Part model, mm, in its own coordinate system. A direction names the side the tool comes from. Give positions to 0.01 mm unless a question says otherwise; leave off trailing zeros. Write each loop counter-clockwise with the first axis right and the second up, starting at its lowest first coordinate (ties: lowest second). Pieces come first, ordered by that corner, then holes. Notation, with made-up numbers: (4.5, 42) - (35.5, 42) arc R18 ccw to (35.5, 67) - close; hole circle Ø3 at (12.25, -6.5). An arc over 180 degrees is marked (long way). Answer as a JSON object with one key per item and string values. Group by question number.
Autodesk Inventor part; units mm, degrees
ref_plane "YZ Plane" through (0, 0, 0) normal (1, 0, 0) x (0, 1, 0)
ref_plane "XZ Plane" through (0, 0, 0) normal (0, 1, 0) x (-1, 0, 0)
ref_plane "XY Plane" through (0, 0, 0) normal (0, 0, 1) x (1, 0, 0)
sketch "Skizze1" plane through (0, 0, 0) normal (0, 1, 0) x (-1, 0, 0)
  line L0 (6.8592, -116.2444) -> (0.8592, -116.2444)
  line L1 (0.8592, -116.2444) -> (0.8592, 8.7556)
  line L2 (6.8592, 8.7556) -> (6.8592, -116.2444)
  line L3 (7.8592, -116.2444) -> (-0.1408, -116.2444)
  line L4 (-0.1408, -116.2444) -> (-0.1408, -106.2444)
  line L5 (-0.1408, -106.2444) -> (7.8592, -106.2444)
  line L6 (7.8592, -106.2444) -> (7.8592, -116.2444)
  line L7 (3.8592, 157.3916) -> (3.8592, -262.6084)
  line L8 (6.8592, 8.7556) -> (0.8592, 8.7556)
  point P0 (0, 0)
  point P1 (0.8592, -106.2444)
  point P2 (6.8592, -106.2444)
  point P3 (6.8592, -116.2444)
  point P4 (3.8592, -116.2444)
  dimension "d1" = 125
  dimension "d9" = 6
  dimension "d25" = 8
  dimension "d26" = 10
  dimension "d27" = 1
extrude "Extrusion1" add sketch "Skizze1" along normal blind 3
sketch "Skizze2" plane through (0, 3, 0) normal (0, 1, 0) x (1, 0, 0)
  line L0 (-3.8592, 111.2444) -> (-6.8592, 111.2444) construction
  line L1 (-3.8592, 111.2444) -> (-0.8592, 111.2444) construction
  line L2 (-0.8592, -8.7556) -> (-0.8592, 106.2444) construction
  line L3 (-6.8592, 106.2444) -> (-6.8592, -8.7556) construction
  line L4 (0.1408, 116.2444) -> (-7.8592, 116.2444)
  point P0 (0, 0)
  point P1 (-0.8592, 16.2444)
  point P2 (-6.8592, 16.2444)
  dimension "d28" = 5
hole "Bohrung1" at (-3.8592, 3, -111.2444) direction (0, -1, 0) diameter 2.459 end through all
sketch "Skizze3" plane through (0.1408, 0, -116.2444) normal (0, 0, -1) x (-1, 0, 0)
  line L0 (4, 0) -> (4, 0.7)
  circle A0 centre (4, 0.7) radius 1.5
  line L1 (0, 0) -> (8, 0)
  point P0 (0.1408, 0)
  dimension "d29" = 3
  dimension "d30" = 0.7
extrude "Extrusion2" add sketch "Skizze3" along normal blind 3
sketch "Skizze4" plane through (0, 0, 0) normal (0, -1, 0) x (1, 0, 0)
  line L0 (-0.8592, 8.7556) -> (-0.8592, -106.2444)
  line L1 (-6.8592, -69.2444) -> (-0.8592, -69.2444)
  line L2 (-0.8592, -69.2444) -> (-0.8592, -29.2444)
  line L3 (-0.8592, -29.2444) -> (-6.8592, -29.2444)
  line L4 (-6.8592, -29.2444) -> (-6.8592, -69.2444)
  point P0 (0, 0)
  point P1 (-0.8592, -69.2444)
  point P2 (-6.8592, -106.2444)
  dimension "d34" = 40
  dimension "d37" = 37
  dimension "d38" = 6
extrude "Extrusion3" add sketch "Skizze4" along normal blind 6
chamfer "Fasen1" distance 40 distance2 4 1 edges at (-3.8592, -6, -29.2444) measured on face at (-4.8592, -6, -42.5778)
properties part number "SchubstangeA" material "PC/ABS-Kunststoff, 3DDruck, PLA"
1) Drop flat-ended pins along their axis: P1, Ø0.6, axis at x = -4.5, y = -1, coming from the +Z side; P2, Ø2, axis at x = -4.5, z = -59, coming from the -Y side; P3, Ø1, axis at x = -1.5, z = -16, coming from the -Y side. Give the stop position or say it passes through.
2) Two-plate mould, pull along Z, no slides. Class faces 5 (the flat face through (-4, 0, -92)), 6 (the flat face through (-4, -1, -29.244)), 7 (the cylindrical face through (-3.913, 1.479, -112.473)), 8 (the flat face through (-0.859, 0, -50)): +Z half, -Z half, draft (parallel to the pull), parting line (faces both ways), or undercut.
3) Which spindle directions (+Z, -Z, +X, -X, +Y, -Y) get a long thin tool onto all of the face, cutting with end or side? Do faces 1 (the flat face through (-7.859, 1, -111)), 2 (the cylindrical face through (-2.36, 0.63, -117.72)), 3 (the flat face through (-4, 0, -10)), 4 (the flat face through (-6.859, 0, -48)). Say none if no direction does.
4) Saw through at A-A (z = -74). List the corners of the cut face in (x, y).
5) Drill centre lines: line 1 along Y through (x, z) = (-1, -5); line 2 along X through (y, z) = (0, -50); line 3 along Z through (x, y) = (-7.5, 2.5). Where is each one in solid material? Low to high. Write a range as from..to.
6) Saw through at B-B (z = -54.5). List the corners of the cut face in (x, y), and give its area (3 significant figures).
Checks:
{
 "1": {"P1": "z = -29.24", "P2": "y = -5.08", "P3": "y = 0"},
 "2": {"face 5": "undercut", "face 6": "+Z half", "face 7": "undercut", "face 8": "draft"},
 "3": {"face 1": "+Z, -Z, -X, +Y, -Y", "face 2": "-Z", "face 3": "+Z, +X, -X, -Y", "face 4": "+Z, -X, +Y, -Y"},
 "4": {"outline": "(-6.86, 0) - (-0.86, 0) - (-0.86, 3) - (-6.86, 3) - close"},
 "5": {"line 1": "0..3", "line 2": "-6.86..-0.86", "line 3": "-116.24..-106.24"},
 "6": {"outline": "(-6.86, -4.53) - (-0.86, -4.53) - (-0.86, 3) - (-6.86, 3) - close", "area": "45.2 mm2"}
}
